The listing builds one solid part. Answer for the finished solid, in the listing's coordinates (mm). Coordinates: 2 decimals unless noted, no trailing zeros. Loops run counter-clockwise (first coordinate to the right, second up) from the corner with the lowest first, then second, coordinate; pieces in that order, holes last. Notation, with made-up numbers: (26, 48) -> (49, 48) arc R15 cw to (49, 55) -> close; hole circle Ø11 at (-19, 68.5). An arc over 180 degrees is marked (long way). Answer in a Markdown table with one row per item.
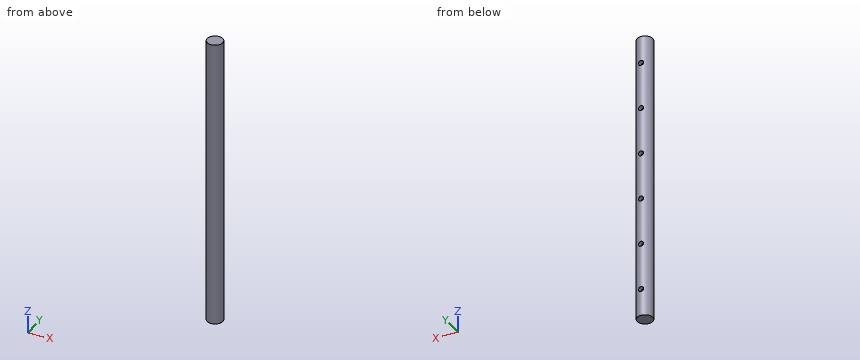
Autodesk Inventor part; units mm, degrees
ref_plane "Work Plane1" through (0, 10, 370) normal (0, 1, 0) x (-1, 0, 0)
ref_plane "YZ Plane" through (0, 0, 0) normal (1, 0, 0) x (0, 1, 0)
ref_plane "XZ Plane" through (0, 0, 0) normal (0, 1, 0) x (-1, 0, 0)
sketch "Sketch1" plane through (0, 0, 0) normal (0, 0, 1) x (1, 0, 0)
  circle A0 centre (0, 0) radius 10
  dimension "d0" = 20
extrude "Extrusion1" add sketch "Sketch1" along normal blind 370
sketch "Sketch2" plane through (0, 0, 370) normal (0, 0, 1) x (1, 0, 0)
  circle A0 centre (0, 0) radius 10
  point P0 (0, 10)
ref_plane "Work Plane1" through (0, 10, 370) normal (0, 1, 0) x (-1, 0, 0)
sketch "Sketch3" plane through (0, 10, 370) normal (0, 1, 0) x (-1, 0, 0)
  line L0 (10, 0) -> (-10, 0)
  line L1 (0, 0) -> (0, -7.8686) construction
  point P0 (0, -370)
  point P1 (0, -35)
  point P2 (0, -95)
  point P3 (0, -155)
  point P4 (0, -215)
  point P5 (0, -275)
  point P6 (0, -335)
  dimension "d3" = 35
  dimension "d6" = 60
hole "Hole1" at (0, 10, 335) at (0, 10, 275) at (0, 10, 215) at (0, 10, 155) at (0, 10, 95) at (0, 10, 35) direction (0, -1, 0) diameter 6.5278 depth 6.35
properties part number "diy-rail_370mm"
Item 1: A cutting plane is placed at A-A, the plane z = 173. Determine the outline of the cut face in (x, y), plus the area to 3 significant figures.
Findings below:
| item | result |
|---|---|
| outline | circle Ø20 at (0, 0) |
| area | 314 mm2 |
Item 2: A cutting plane is placed at C-C, the plane z = 275. Determine the outline of the cut face in (x, y), plus the area to 3 significant figures.
Findings below:
| item | result |
|---|---|
| outline | (-3.26, 3.65) -> (-3.26, 9.45) arc R10 ccw (long way) to (3.26, 9.45) -> (3.26, 3.65) -> close |
| area | 274 mm2 |
Item 3: A cutting plane is placed at B-B, the plane y = -5.75. Determine the outline of the cut face in (x, z), plus the area to 3 significant figures.
Findings below:
| item | result |
|---|---|
| outline | (-8.18, 0) -> (8.18, 0) -> (8.18, 370) -> (-8.18, 370) -> close |
| area | 6,050 mm2 |
Item 4: Find the intervals of material crossed by probe 1 along X at (y, z) = (9, 97); probe 2 along X at (y, z) = (7.5, 275); probe 3 along Y at (x, z) = (0, 278), in increasing order.
Findings below:
| item | result |
|---|---|
| probe 1 | x = -4.36 to -2.58, 2.58 to 4.36 |
| probe 2 | x = -6.61 to -3.26, 3.26 to 6.61 |
| probe 3 | y = -10 to 3.65 |
Item 5: Flat-ended cylindrical pins translate along their axes: pin 1 Ø2 at (y, z) = (7, 141) entering from -X; pin 2 Ø1.5 at (y, z) = (-2.5, 317) entering from -X; pin 3 Ø4 at (x, z) = (7.5, 146) entering from +Y. Find the tip coordinate at first contact, or state that the pin passes through.
Findings below:
| item | result |
|---|---|
| pin 1 | stops at x = -8 |
| pin 2 | stops at x = -9.85 |
| pin 3 | stops at y = 8.35 |
